Model file for the job. Use its own axes, mm. A direction names the side the tool comes from. Round coordinates to 2 decimals unless told otherwise and drop trailing zeros. Order: outer loops, then holes, each group sorted by start corner. A loop starts at its lowest first (then second) coordinate and runs counter-clockwise, first axis right, second up. Notation, with made-up numbers: (50, -0.5) - (105, -0.5) arc R33 cw to (105, 38.5) - close; hole circle Ø7 at (-9, 5.5). An arc over 180 degrees is marked (long way). Answer as CSV lines item,"result". Start each with the question number.
1. Pull direction Y, two halves, no side cores. Call faces 1 (the face through (-69.85, -1, 34)), 2 (the face through (-54.468, -33.902, 24.625)), 3 (the face through (54, -25.4, 25)): released by +Y, released by -Y, zero draft, split by the parting line, or undercut.
2. Band-saw the part on C-C on z = 33.5. State how many separate pieces and enclosed holes the cut face has, then the cut area to 3 significant figures.
3. Pin check, flat tips, straight feed: pin 1 Ø1 at (x, z) = (7.5, 28) entering from -Y; pin 2 Ø7 at (x, z) = (58, 26.5) entering from +Y; pin 3 Ø4 at (x, z) = (-50, 25) entering from +Y; pin 4 Ø6 at (x, y) = (-30.5, -10.5) entering from -Z. Stop position of each tip, or through.
4. Wall check: line 1 along X through (y, z) = (22.5, 33.5); line 2 along X through (y, z) = (6.5, 30); line 3 along Z through (x, y) = (59.5, 24). Give the ranges that are in metal, low to high. Write a range as [from, to].
5. Band-saw the part on D-D on x = 0. List the corners of the cut face in (y, z).
6. 3-axis set-ups, long thin cutter, end or side, ignore diameter. For faces 4 (the face through (24.64, 23, 33)), 5 (the face through (54, -42.672, 25)), 6 (the face through (64.77, -34, 26)): which of +Z, -Z, +X, -X, +Y, -Y reach the whole face in a straight line?
7. Band-saw the part on A-A on y = 58.42. List the corners of the cut face in (x, z), then the cut area to 3 significant figures.
```python
from build123d import *

# Parameters (mm, degrees)
BOX_W                = 40.39
BOX_H                = 86.36
BOX_DEPTH            = 25.4
SKETCH045_W          = 139.7
SKETCH045_H          = 127
PAD022_DEPTH         = 3.81
SKETCH046_W          = 133.096
SKETCH046_H          = 120.396
PAD023_DEPTH         = 2.16
SKETCH013_R          = 1.5621
SKETCH013_R_2        = 1.651
POCKET019_DEPTH      = 5.971
SKETCH047_W          = 20.32
SKETCH047_H          = 17.272
PAD024_DEPTH         = 12.7
SKETCH048_R          = 12.3825
POCKET020_DEPTH      = 69.851
POCKET020_DEPTH_BACK = 69.851


with BuildPart() as top_removal:
    # Box → Box (new body)
    with BuildSketch(Plane(origin=(-15.75, -16.89, 13.87), x_dir=(1, 0, 0), z_dir=(0, 0, 1))):
        with Locations((20.195, 43.18)):
            Rectangle(BOX_W, BOX_H)
    extrude(amount=BOX_DEPTH)


with BuildPart() as top_cover:
    # Sketch045 → Pad022 (new body)
    with BuildSketch(Plane.XY.offset(31.75)):
        Rectangle(SKETCH045_W, SKETCH045_H)
    extrude(amount=PAD022_DEPTH)

    # Sketch046 (on Face5 of Pad022) → Pad023 (join)
    with BuildSketch(Plane(origin=(0, 0, 31.75), x_dir=(1, 0, 0), z_dir=(0, 0, -1))):
        Rectangle(SKETCH046_W, SKETCH046_H)
    extrude(amount=PAD023_DEPTH)

    # Sketch013 (on Face5 of Pad023) → Pocket019 (cut, through all)
    with BuildSketch(Plane.XY.offset(35.56)):
        with Locations((64.7827376585, 58.42)):
            Circle(SKETCH013_R)
        with Locations((64.7827376585, 0)):
            Circle(SKETCH013_R)
        with Locations((64.7827376585, -58.42)):
            Circle(SKETCH013_R)
        with Locations((0, 58.42)):
            Circle(SKETCH013_R)
        with Locations((-64.7827376585, 58.42)):
            Circle(SKETCH013_R)
        with Locations((-64.7827376585, 0.043989)):
            Circle(SKETCH013_R)
        with Locations((-64.7827376585, -58.42)):
            Circle(SKETCH013_R)
        with Locations((0, -58.42)):
            Circle(SKETCH013_R)
        with Locations((-27.313105, 2.676934)):
            Circle(SKETCH013_R_2)
        with Locations((-27.313105, -13.325066)):
            Circle(SKETCH013_R_2)
    extrude(amount=-POCKET019_DEPTH, mode=Mode.SUBTRACT)

    # Sketch047 (on Face21 of Pocket019) → Pad024 (join)
    with BuildSketch(Plane(origin=(0, 0, 29.59), x_dir=(1, 0, 0), z_dir=(0, 0, -1))):
        with Locations((-54.61, 34.036)):
            Rectangle(SKETCH047_W, SKETCH047_H)
        with Locations((54.61, 34.036)):
            Rectangle(SKETCH047_W, SKETCH047_H)
    extrude(amount=PAD024_DEPTH)

    # Sketch048 → Pocket020 (cut, two sides)
    with BuildSketch(Plane.YZ) as pocket020_sk:
        with Locations((-34.036, 12.2428)):
            Circle(SKETCH048_R)
    extrude(amount=-POCKET020_DEPTH, mode=Mode.SUBTRACT)
    extrude(pocket020_sk.sketch, amount=POCKET020_DEPTH_BACK, mode=Mode.SUBTRACT)

    # Cut: cut top_removal
    add(top_removal.part, mode=Mode.SUBTRACT)


solid = top_cover.part
```
Reply:
1,face 1,"zero draft"
1,face 2,"undercut"
1,face 3,"released by +Y"
2,separate pieces,"1"
2,enclosed holes,"9"
2,area,"14,400 mm2"
3,pin 1,"passes through"
3,pin 2,"stops at y = 60.2"
3,pin 3,"stops at y = -25.4"
3,pin 4,"stops at z = 29.59"
4,line 1,"x = [-69.85, -15.75], [24.64, 69.85]"
4,line 2,"x = [-66.55, -15.75], [24.64, 66.55]"
4,line 3,"z = [29.59, 35.56]"
5,outline,"(-63.5, 31.75) - (-60.2, 31.75) - (-60.2, 29.59) - (-59.98, 29.59) - (-59.98, 35.56) - (-63.5, 35.56) - close; (-56.86, 29.59) - (-16.89, 29.59) - (-16.89, 35.56) - (-56.86, 35.56) - close"
6,face 4,"+Z, -Z, +Y"
6,face 5,"-Z, +X, -X, -Y"
6,face 6,"-Z, +X, +Y, -Y"
7,outline,"(-69.85, 31.75) - (-66.55, 31.75) - (-66.55, 29.59) - (-66.34, 29.59) - (-66.34, 35.56) - (-69.85, 35.56) - close; (-63.22, 29.59) - (-15.75, 29.59) - (-15.75, 35.56) - (-63.22, 35.56) - close; (24.64, 29.59) - (63.22, 29.59) - (63.22, 35.56) - (24.64, 35.56) - close; (66.34, 29.59) - (66.55, 29.59) - (66.55, 31.75) - (69.85, 31.75) - (69.85, 35.56) - (66.34, 35.56) - close"
7,area,"541 mm2"
